```python
from build123d import *

# Parameters (mm, degrees)
SKETCH1_W           = 4
SKETCH1_H           = 5
BOSS_EXTRUDE1_DEPTH = 2
SKETCH2_W           = 4
SKETCH2_H           = 2
BOSS_EXTRUDE2_DEPTH = 2
BOSS_EXTRUDE3_DEPTH = 2
BOSS_EXTRUDE4_DEPTH = 5
CUT_EXTRUDE1_DEPTH  = 5


with BuildPart() as part:
    # Sketch1 → Boss-Extrude1 (new body)
    with BuildSketch(Plane.XY):
        Rectangle(SKETCH1_W, SKETCH1_H)
    extrude(amount=BOSS_EXTRUDE1_DEPTH)

    # Sketch2 → Boss-Extrude2 (add)
    with BuildSketch(Plane.XY.offset(2)):
        with Locations((0, -1.5)):
            Rectangle(SKETCH2_W, SKETCH2_H)
    extrude(amount=BOSS_EXTRUDE2_DEPTH)

    # Sketch3 → Boss-Extrude3 (add)
    with BuildSketch(Plane(origin=(0, -0.5, 0), x_dir=(1, 0, 0), z_dir=(0, 1, 0))):
        Polygon((2, -4), (4, -2), (2, -2), align=None)
    extrude(amount=-BOSS_EXTRUDE3_DEPTH)

    # Sketch4 → Boss-Extrude4 (add)
    with BuildSketch(Plane(origin=(0, 2.5, 0), x_dir=(1, 0, 0), z_dir=(0, 1, 0))):
        Polygon((2, 0), (4, -2), (1.353311903, -2), align=None)
    extrude(amount=-BOSS_EXTRUDE4_DEPTH)

    # Sketch5 → Cut-Extrude1 (cut)
    with BuildSketch(Plane(origin=(0, 2.5, 0), x_dir=(1, 0, 0), z_dir=(0, 1, 0))):
        Polygon((-2, -2), (0, -2), (2, 0), (-2, 0), align=None)
    extrude(amount=-CUT_EXTRUDE1_DEPTH, mode=Mode.SUBTRACT)


solid = part.part
```
Part model, mm, in its own coordinate system. A direction names the side the tool comes from. Coordinates: 2 decimals unless noted, no trailing zeros. Loops run counter-clockwise (first coordinate to the right, second up) from the corner with the lowest first, then second, coordinate; pieces in that order, holes last. Notation, with made-up numbers: (55.25, 83) - (66.25, 83) arc R22 ccw to (66.25, 93) - close; hole circle Ø2 at (-25, -14). An arc over 180 degrees is marked (long way). Write item = value, one per line. Start each with the question number.
Item 1: Cut at B-B, the plane z = 2.3. Give the cut face in (x, y).
Item 2: Flat gauge pins, fed straight in: pin 1 Ø2 at (x, z) = (0, 3.5) entering from +Y; pin 2 Ø1.6 at (x, y) = (-1, -1.5) entering from -Z; pin 3 Ø2 at (x, y) = (2.5, -0.5) entering from -Z. Where does each tip first touch, or does it go through?
Item 3: 3-axis set-ups, long thin cutter, end or side, ignore diameter. For faces 1 (the flat face through (1, -2.5, 2)), 2 (the flat face through (-1, -1, 2)), 3 (the flat face through (0, -0.5, 3)): which of +Z, -Z, +X, -X, +Y, -Y reach the whole face in a straight line?
Item 4: Cut at A-A, the plane x = 0.85. Give the cut face in (y, z), and give its area (3 significant figures).
Item 5: Wall check: L1, parallel to Y at x = 2.2, z = 2.2; L2, parallel to Z at x = 2.25, y = 0.9; L3, parallel to X at y = -2.05, z = 3.6. Give the ranges that are in metal, low to high. Write a range as from..to.
Item 6: Cut at D-D, the plane x = 3.6. Give the cut face in (y, z).
Item 7: Cut at C-C, the plane y = 2. Give the cut face in (x, z), and give its area (3 significant figures).
The answers:
q1.outline = (-2, -2.5) - (3.7, -2.5) - (3.7, -0.5) - (-2, -0.5) - close
q2.pin_1 = -0.5
q2.pin_2 = 2
q2.pin_3 = 0
q3.face_1 = +Z, -Z, +X, -X, -Y
q3.face_2 = -Z, -X, +Y, -Y
q3.face_3 = +Z, +X, -X, +Y
q4.outline = (-2.5, 1.15) - (2.5, 1.15) - (2.5, 2) - (-0.5, 2) - (-0.5, 4) - (-2.5, 4) - close
q4.area = 8.25 mm2
q5.L1 = -2.5..-0.5
q5.L2 = 0.25..2
q5.L3 = -2..2.4
q6.outline = (-2.5, 1.6) - (2.5, 1.6) - (2.5, 2) - (-0.5, 2) - (-0.5, 2.4) - (-2.5, 2.4) - close
q7.outline = (0, 2) - (2, 0) - (4, 2) - close
q7.area = 4.00 mm2
